from build123d import *

# Parameters (mm, degrees)
REVOLVE2_ANGLE     = 270
SKETCH5_R          = 3.175
CUT_EXTRUDE1_DEPTH = 46.023434974
FILLET1_R          = 2.54
FILLET2_R          = 2.54


with BuildPart() as part:
    # Sketch1 → Revolve2 (revolve)
    with BuildSketch(Plane(origin=(0, 0, 0), x_dir=(0, 0, -1), z_dir=(1, 0, 0))):
        Polygon((22.479, 35.498434974), (22.479, 45.023434974), (25.654, 45.023434974), (25.654, 0.573434974), (22.479, 0.573434974), (22.479, 32.323434974), (6.35, 32.323434974), (6.35, 0.573434974), (3.175, 0.573434974), (3.175, 45.023434974), (6.35, 45.023434974), (6.35, 35.498434974), align=None)
    revolve(axis=Axis((0, 45.023434974, 0), (0, -1, 0)), revolution_arc=REVOLVE2_ANGLE)

    # Sketch5 → Cut-Extrude1 (cut, through all)
    with BuildSketch(Plane(origin=(0, 0, 0), x_dir=(1, 0, 0), z_dir=(0, 1, 0))):
        with Locations((0, 12.7)):
            Circle(SKETCH5_R)
    extrude(amount=CUT_EXTRUDE1_DEPTH, mode=Mode.SUBTRACT)

    # Fillet1
    fillet1_edges = [part.edges().sort_by_distance(p)[0] for p in [
        (15.895053334, 32.323434974, 15.895053334),
        (4.490128061, 32.323434974, 4.490128061),
    ]]
    fillet(fillet1_edges, radius=FILLET1_R)

    # Fillet2
    fillet2_edges = [part.edges().sort_by_distance(p)[0] for p in [
        (4.490128061, 35.498434974, 4.490128061),
        (15.895053334, 35.498434974, 15.895053334),
    ]]
    fillet(fillet2_edges, radius=FILLET2_R)


solid = part.part
Work out the finished part from the listing and answer in its coordinate system (mm). A direction names the side the tool comes from. Give positions to 0.01 mm unless a question says otherwise; leave off trailing zeros. Write each loop counter-clockwise with the first axis right and the second up, starting at its lowest first coordinate (ties: lowest second). Pieces come first, ordered by that corner, then holes. Notation, with made-up numbers: (62, -8) - (70, -8) arc R22 cw to (70, 30) - close; hole circle Ø6 at (59.5, 87.5). An arc over 180 degrees is marked (long way). One line per item, written item: value. Start each with the question number.
1. For a pull along X with two mould halves and no side action, classify faces 4 (the flat face through (0, 23, -23)), 5 (the flat face through (15, 45.023, 17)), 6 (the cylindrical face through (2.32, 23.11, 2.17)) as +X half, -X half, draft (parallel to the pull), parting line (faces both ways), or undercut.
2. For faces 1 (the flat face through (5, 35.498, 9)), 2 (the cylindrical face through (4.636, 14.974, 4.34)), 3 (the flat face through (0, 23, -5)), determine the directions among +Z, -Z, +X, -X, +Y, -Y from which every point of the face is accessible in a straight line to the end or side of a thin tool.
3. Given pin 1 (8 mm diameter, centred on x = 16, y = 27, fed in from +Z); pin 2 (6 mm diameter, centred on x = -2, y = 15.5, fed in from +Z); pin 3 (12 mm diameter, centred on y = 25.5, z = 14, fed in from +X); pin 4 (3 mm diameter, centred on y = 31, z = -19, fed in from -X), each flat-ended and moving along its own axis, determine where each tip first touches the part or whether it passes through.
4. Consider probe 1 along Y at (x, z) = (11.5, -3.5); probe 2 along Z at (x, y) = (-0.5, 11.5); probe 3 along X at (y, z) = (21, 10). Determine where each line is inside the solid, lowest interval first.
5. Find section A-A (y = 15.5). Write down the section's boundary in (x, z) (3 decimals).
Geometry results:
1. face 4: -X half
1. face 5: draft
1. face 6: undercut
2. face 1: +Y
2. face 2: -Y
2. face 3: -Z, -X, +Y, -Y
3. pin 1: z = 22.67
3. pin 2: z = 25.65
3. pin 3: x = 24.37
3. pin 4: x = 0
4. probe 1: 32.32 to 35.5
4. probe 2: 3.14 to 6.33, 22.47 to 25.65
4. probe 3: -23.62 to -20.13, 20.13 to 23.62
5. outline: (-25.654, 0) - (-22.479, 0) arc R22.479 cw (long way) to (0, -22.479) - (0, -25.654) arc R25.654 ccw (long way) to start; (-6.35, 0) - (-3.175, 0) arc R3.175 cw (long way) to (0, -3.175) - (0, -6.35) arc R6.35 ccw (long way) to start
